from build123d import *

# Parameters (mm, degrees)
SKETCH1_W           = 50
SKETCH1_H           = 30
BOSS_EXTRUDE2_DEPTH = 10
BOSS_EXTRUDE3_DEPTH = 10
BOSS_EXTRUDE4_DEPTH = 10
SKETCH6_R           = 7.353544845
CUT_EXTRUDE1_DEPTH  = 10


with BuildPart() as part:
    # Sketch1 → Boss-Extrude2 (new body)
    with BuildSketch(Plane.XY):
        with Locations((0, -15)):
            Rectangle(SKETCH1_W, SKETCH1_H)
    extrude(amount=BOSS_EXTRUDE2_DEPTH)

    # Sketch4 → Boss-Extrude3 (add)
    with BuildSketch(Plane.XY.offset(10)):
        with BuildLine():
            Line((25, 0), (25, -30))
            ThreePointArc((25, -30), (40, -15), (25, 0))
        make_face()
    extrude(amount=-BOSS_EXTRUDE3_DEPTH)

    # Sketch5 → Boss-Extrude4 (add)
    with BuildSketch(Plane.XY.offset(10)):
        with BuildLine():
            Line((-25, 0), (-25, -30))
            ThreePointArc((-25, -30), (-40, -15), (-25, 0))
        make_face()
    extrude(amount=-BOSS_EXTRUDE4_DEPTH)

    # Sketch6 → Cut-Extrude1 (cut)
    with BuildSketch(Plane.XY.offset(10)):
        with Locations((-25, -15)):
            Circle(SKETCH6_R)
        with Locations(Location((25, -15, 0), (0, 0, 180))):
            Circle(SKETCH6_R)
    extrude(amount=-CUT_EXTRUDE1_DEPTH, mode=Mode.SUBTRACT)


solid = part.part
For this review, take the finished solid that the model builds, in its own axes (mm). Coordinates: 2 decimals unless noted, no trailing zeros. Order: outer loops, then holes, each group sorted by start corner. A loop starts at its lowest first (then second) coordinate and runs counter-clockwise, first axis right, second up. Notation, with made-up numbers: (4.5, 77) - (31.5, 77) arc R19 ccw to (31.5, 98) - close; hole circle Ø2 at (4.5, 32.5). An arc over 180 degrees is marked (long way). Answer as CSV lines item,"result". Start each with the question number.
1) To check wall thickness, follow line 1 along Y through (x, z) = (25, 4.5); line 2 along X through (y, z) = (-21.5, 6.5); line 3 along X through (y, z) = (-11.5, 6.5). State the ranges of each line that lie inside material, in increasing order. Write a range as [from, to].
2) Add section C-C (z = 2.5). State the section outline as (x, y) points.
3) Add section D-D (y = -10). State the section outline as (x, z) points, then the cut area to 3 significant figures.
4) Add section A-A (y = -15). State the section outline as (x, z) points, then the cut area to 3 significant figures.
5) Insertion check: P1, Ø4, axis at y = -8.5, z = 4, coming from the -X side; P2, Ø3, axis at y = -10.5, z = 6.5, coming from the -X side; P3, Ø1.5, axis at y = -9, z = 1.5, coming from the -X side. Each pin has a flat end and moves straight along its axis. Give the tip position at first contact, or say it passes through.
6) Draft analysis for pull direction X (two halves, no side actions). For faces 1 (the cylindrical face through (40, -15, 5)), 2 (the cylindrical face through (17.986, -17.209, 5.07)), 3 (the flat face through (1, -15, 0)), 4 (the cylindrical face through (-17.986, -12.791, 5.07)), state which applies: +X half, -X half, draft (parallel to the pull), parting line (faces both ways), or undercut.
7) Add section B-B (x = 20.5). State the section outline as (y, z) points.
Result:
1,line 1,"[-30, -22.35], [-7.65, 0]"
1,line 2,"[-38.52, -28.44], [-21.56, 21.56], [28.44, 38.52]"
1,line 3,"[-39.59, -31.47], [-18.53, 18.53], [31.47, 39.59]"
2,outline,"(-25, -30) - (25, -30) arc R15 ccw to (25, 0) - (-25, 0) arc R15 ccw to start; hole circle Ø14.71 at (-25, -15); hole circle Ø14.71 at (25, -15)"
3,outline,"(-39.14, 0) - (-30.39, 0) - (-30.39, 10) - (-39.14, 10) - close; (-19.61, 0) - (19.61, 0) - (19.61, 10) - (-19.61, 10) - close; (30.39, 0) - (39.14, 0) - (39.14, 10) - (30.39, 10) - close"
3,area,"567 mm^2"
4,outline,"(-40, 0) - (-32.35, 0) - (-32.35, 10) - (-40, 10) - close; (-17.65, 0) - (17.65, 0) - (17.65, 10) - (-17.65, 10) - close; (32.35, 0) - (40, 0) - (40, 10) - (32.35, 10) - close"
4,area,"506 mm^2"
5,P1,"x = -39.31"
5,P2,"x = -39.7"
5,P3,"x = -39.05"
6,face 1,"+X half"
6,face 2,"undercut"
6,face 3,"draft"
6,face 4,"undercut"
7,outline,"(-30, 0) - (-20.82, 0) - (-20.82, 10) - (-30, 10) - close; (-9.18, 0) - (0, 0) - (0, 10) - (-9.18, 10) - close"
